```python
from build123d import *

# Parameters (mm, degrees)
F0_W      = 85
F0_H      = 15
F0_R      = 2.6
F1_DEPTH  = 5
F3_DEPTH  = 2.5
F4_R      = 7
F5_R      = 0.8
F6_DEPTH  = 2.5
F7_W      = 5
F7_H      = 15
F8_DEPTH  = 16
F10_D     = 2.5
F10_DEPTH = 8
F10_TIP   = 0.7510757738
F11_W     = 2.8
F11_H     = 5.2
F12_DEPTH = 33
F13_W     = 26
F13_H     = 7
F14_DEPTH = 15
F15_R     = 1
F16_W     = 4.5
F16_H     = 4.5
F17_DEPTH = 5


with BuildPart() as f1:
    # F0 (on Front) → F1 (new body)
    with BuildSketch(Plane.XZ):
        with Locations((42.5, 0)):
            Rectangle(F0_W, F0_H)
        with Locations((65, 0)):
            Circle(F0_R, mode=Mode.SUBTRACT)
    extrude(amount=-F1_DEPTH)

    # F2 (on face) → F3 (cut)
    with BuildSketch(Plane(origin=(0, 5, 0), x_dir=(-1, 0, 0), z_dir=(0, 1, 0))):
        with BuildLine():
            Line((-81.8847875997, -2.6724405518), (-69.1919565837, -4.5))
            ThreePointArc((-69.1919565837, -4.5), (-65, -6.15), (-60.8080434163, -4.5))
            Line((-60.8080434163, -4.5), (-48.1152124003, -2.6724405518))
            ThreePointArc((-48.1152124003, -2.6724405518), (-45.8, 0), (-48.1152124003, 2.6724405518))
            Line((-48.1152124003, 2.6724405518), (-60.8080434163, 4.5))
            ThreePointArc((-60.8080434163, 4.5), (-65, 6.15), (-69.1919565837, 4.5))
            Line((-69.1919565837, 4.5), (-81.8847875997, 2.6724405518))
            ThreePointArc((-81.8847875997, 2.6724405518), (-84.2, 0), (-81.8847875997, -2.6724405518))
        make_face()
    extrude(amount=-F3_DEPTH, mode=Mode.SUBTRACT)

    # F4
    f4_edges = [f1.edges().sort_by_distance(p)[0] for p in [
        (85, 2.5, 7.5),
        (85, 2.5, -7.5),
        (0, 2.5, 7.5),
        (0, 2.5, -7.5),
    ]]
    fillet(f4_edges, radius=F4_R)

    # F5 (on face) → F6 (cut, through all)
    with BuildSketch(Plane(origin=(0, 2.5, 0), x_dir=(-1, 0, 0), z_dir=(0, 1, 0))):
        with Locations((-81.5, 0)):
            Circle(F5_R)
        with Locations((-78.5, 0)):
            Circle(F5_R)
        with Locations((-75.5, 0)):
            Circle(F5_R)
        with Locations((-72.5, 0)):
            Circle(F5_R)
        with Locations((-57.5, 0)):
            Circle(F5_R)
        with Locations((-54.5, 0)):
            Circle(F5_R)
        with Locations((-51.5, 0)):
            Circle(F5_R)
        with Locations((-48.5, 0)):
            Circle(F5_R)
    extrude(amount=-F6_DEPTH, mode=Mode.SUBTRACT)

    # F7 (on face) → F8 (join)
    with BuildSketch(Plane(origin=(0, 5, 0), x_dir=(-1, 0, 0), z_dir=(0, 1, 0))):
        with Locations((-33, 0)):
            Rectangle(F7_W, F7_H)
        with BuildLine():
            Line((-7, 7.5), (-7.5, 7.5))
            Line((-7.5, 7.5), (-7.5, -7.5))
            Line((-7.5, -7.5), (-7, -7.5))
            ThreePointArc((-7, -7.5), (-4.6055604551, -7.0777396776), (-2.5, -5.8619026474))
            Line((-2.5, -5.8619026474), (-2.5, 5.8619026474))
            ThreePointArc((-2.5, 5.8619026474), (-4.6055604551, 7.0777396776), (-7, 7.5))
        make_face()
    extrude(amount=F8_DEPTH)

    # F10
    with Locations(Plane(origin=(0, 21, 0), x_dir=(-1, 0, 0), z_dir=(0, 1, 0))):
        with Locations((-32.85, 0), (-5.15, 0)):
            Hole(F10_D / 2, depth=F10_DEPTH)
            with Locations((0, 0, -(F10_DEPTH + F10_TIP / 2))):  # 118° drill point
                Cone(0, F10_D / 2, F10_TIP, mode=Mode.SUBTRACT)

    # F11 (on face) → F12 (cut, through all)
    with BuildSketch(Plane(origin=(2.5, 0, 0), x_dir=(0, -1, 0), z_dir=(-1, 0, 0))):
        with Locations((-17.6, 0)):
            Rectangle(F11_W, F11_H)
    extrude(amount=-F12_DEPTH, mode=Mode.SUBTRACT)

    # F13 (on face) → F14 (cut, through all)
    with BuildSketch(Plane(origin=(0, 0, -7.5), x_dir=(1, 0, 0), z_dir=(0, 0, -1))):
        with Locations((19, -8.5)):
            Rectangle(F13_W, F13_H)
    extrude(amount=-F14_DEPTH, mode=Mode.SUBTRACT)

    # F15
    f15_edges = [f1.edges().sort_by_distance(p)[0] for p in [
        (32, 12, 0),
        (6, 12, 0),
    ]]
    fillet(f15_edges, radius=F15_R)

    # F16 (on face) → F17 (cut, through all)
    with BuildSketch(Plane.YZ.offset(35.5)):
        with Locations((9.75, 0)):
            Rectangle(F16_W, F16_H)
    extrude(amount=-F17_DEPTH, mode=Mode.SUBTRACT)


solid = f1.part
```
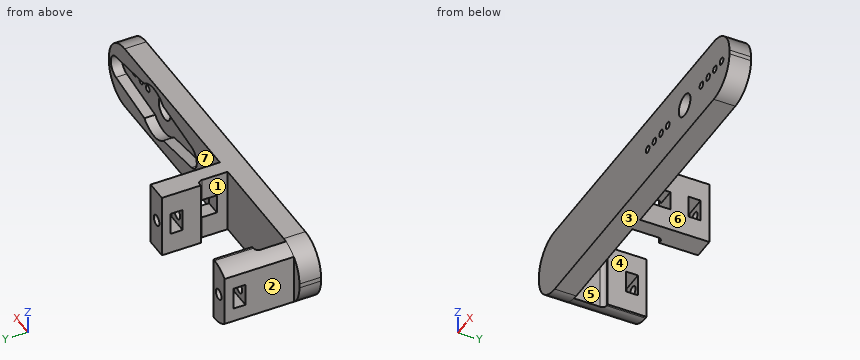
Could you check a few things on this model? Use its own coordinates, in mm. Face numbers are marked on the shaded views. A direction names the side the tool comes from. Round coordinates to 2 decimals unless told otherwise and drop trailing zeros. Write each loop counter-clockwise with the first axis right and the second up, starting at its lowest first coordinate (ties: lowest second). Pieces come first, ordered by that corner, then holes.
(1) Suppose I cut it at C-C on z = -3.5. Write out the boundary of the cut face in (x, y), and give its area (3 significant figures).
Findings below:
outline: (0.68, 0) - (84.32, 0) - (84.32, 5) - (76.14, 5) - (76.14, 2.5) - (53.86, 2.5) - (53.86, 5) - (35.5, 5) - (35.5, 21) - (30.5, 21) - (30.5, 12) - (31, 12) arc R1 cw to (32, 11) - (32, 5) - (6, 5) - (6, 11) arc R1 cw to (7, 12) - (7.5, 12) - (7.5, 21) - (2.5, 21) - (2.5, 5) - (0.68, 5) - close
area: 502 mm2
(2) For pin 1 (2.5 mm diameter, centred on x = 34, z = 2.5, fed in from -Y); pin 2 (1 mm diameter, centred on y = 6, z = -4, fed in from -X); pin 3 (3.5 mm diameter, centred on x = 68, z = 0, fed in from +Y); pin 4 (2 mm diameter, centred on y = 18, z = -6, fed in from +X), each with a flat end and sliding along its axis, tell me the tip position at first contact or that it passes through.
Findings below:
pin 1: stops at y = 0
pin 2: stops at x = 2.5
pin 3: stops at y = 2.5
pin 4: stops at x = 35.5
(3) Thinking about a two-plate mould opening in Y: for the marked faces 5, 6 and 7, which applies, +Y half, -Y half, draft (parallel to the pull), parting line (faces both ways), or undercut?
Findings below:
face 5: undercut
face 6: draft
face 7: +Y half
(4) If I drill on probe 1 along X at (y, z) = (16, 0); probe 2 along X at (y, z) = (17.25, -6); probe 3 along X at (y, z) = (13, 5.5), over which ranges is the centre line in solid material (lowest first)?
Findings below:
probe 1: x = 2.5 to 3.9, 6.4 to 7.5, 30.5 to 31.6, 34.1 to 35.5
probe 2: x = 2.67 to 7.5, 30.5 to 35.5
probe 3: x = 2.5 to 7.5, 30.5 to 35.5
(5) Suppose I cut it at D-D on x = 51.5. Write out the boundary of the cut face in (y, z), and give its area (3 significant figures).
Findings below:
outline: (0, -7.5) - (5, -7.5) - (5, -3.16) - (2.5, -3.16) - (2.5, -0.8) - (0, -0.8) - close; (0, 0.8) - (2.5, 0.8) - (2.5, 3.16) - (5, 3.16) - (5, 7.5) - (0, 7.5) - close
area: 55.2 mm2
(6) Which directions (+Z, -Z, +X, -X, +Y, -Y) give clear straight access to the entire face, cutting with the end or side of a thin tool? Please do the marked faces 1, 2, 3 and 4.
Findings below:
face 1: +Z, -Z
face 2: +Z, -Z, -X, +Y
face 3: -Z, +X, -X, +Y, -Y
face 4: +Z, -Z, +Y
(7) Suppose I cut it at B-B on y = 17. Write out the boundary of the cut face in (x, z).
Findings below:
outline: (2.5, -5.86) arc R7 ccw to (7, -7.5) - (7.5, -7.5) - (7.5, -2.6) - (2.5, -2.6) - close; (2.5, 2.6) - (7.5, 2.6) - (7.5, 7.5) - (7, 7.5) arc R7 ccw to (2.5, 5.86) - close; (30.5, -7.5) - (35.5, -7.5) - (35.5, -2.6) - (30.5, -2.6) - close; (30.5, 2.6) - (35.5, 2.6) - (35.5, 7.5) - (30.5, 7.5) - close
(8) Suppose I cut it at A-A on x = 65. Write out the boundary of the cut face in (y, z).
Findings below:
outline: (0, -7.5) - (5, -7.5) - (5, -6.15) - (2.5, -6.15) - (2.5, -2.6) - (0, -2.6) - close; (0, 2.6) - (2.5, 2.6) - (2.5, 6.15) - (5, 6.15) - (5, 7.5) - (0, 7.5) - close
